from build123d import *

# Parameters (mm, degrees)
SKETCH_1_R               = 11
SKETCH_1_R_2             = 4
EXTRUDE_1_DEPTH          = 7
SKETCH_2_R               = 12
SKETCH_2_R_2             = 10
CUT_EXTRUDE_1_DEPTH      = 0.5
CUT_EXTRUDE_1_DEPTH_BACK = 0.5


with BuildPart() as part:
    # 草图1 → 凸台-拉伸1 (new body)
    with BuildSketch(Plane(origin=(0, 0, 0), x_dir=(1, 0, 0), z_dir=(0, 1, 0))):
        Circle(SKETCH_1_R)
        Circle(SKETCH_1_R_2, mode=Mode.SUBTRACT)
    extrude(amount=EXTRUDE_1_DEPTH)

    # 草图2 → 切除-拉伸1 (cut, two sides)
    with BuildSketch(Plane(origin=(0, 3.5, 0), x_dir=(1, 0, 0), z_dir=(0, 1, 0))) as cut_extrude_1_sk:
        Circle(SKETCH_2_R)
        Circle(SKETCH_2_R_2, mode=Mode.SUBTRACT)
    extrude(amount=CUT_EXTRUDE_1_DEPTH, mode=Mode.SUBTRACT)
    extrude(cut_extrude_1_sk.sketch, amount=-CUT_EXTRUDE_1_DEPTH_BACK, mode=Mode.SUBTRACT)


solid = part.part
Model file for the job. Use its own axes, mm. A direction names the side the tool comes from. Give positions to 0.01 mm unless a question says otherwise; leave off trailing zeros. Write each loop counter-clockwise with the first axis right and the second up, starting at its lowest first coordinate (ties: lowest second). Pieces come first, ordered by that corner, then holes. Notation, with made-up numbers: M -38,-12 L 12,-12 A28 cw 12,25 Z; hole C 32.25,85.5 d10. An arc over 180 degrees is marked long. One line per item, written item: value. Start each with the question number.
Q1. Saw through at A-A, the plane x = 0. Write the cut outline in (y, z), plus the area to 3 significant figures.
Q2. Saw through at B-B, the plane z = 0. Write the cut outline in (x, y).
Q3. Two-plate mould, pull along X, no slides. Class faces 1 (the flat face through (0, 7, 5)), 2 (the cylindrical face through (-2.38, 1.48, 10.74)), 3 (the cylindrical face through (-0.867, 3.451, 3.905)): +X half, -X half, draft (parallel to the pull), parting line (faces both ways), or undercut.
Q4. Saw through at C-C, the plane y = 2. Write the cut outline in (x, z).
Q5. 3-axis set-ups, long thin cutter, end or side, ignore diameter. For faces 4 (the cylindrical face through (-2.38, 5.48, 10.74)), 5 (the flat face through (2, 4, 10)): which of +Z, -Z, +X, -X, +Y, -Y reach the whole face in a straight line?
Q6. Probe probe 1 along X at (y, z) = (2.75, 0); probe 2 along X at (y, z) = (3.5, 0); probe 3 along Y at (x, z) = (2.75, -10). List the from-to ranges inside material, lowest first. Write a range as [from, to].
Q7. Drop flat-ended pins along their axis: pin 1 Ø11 at (x, z) = (0, 0.5) entering from +Y; pin 2 Ø1 at (x, y) = (3.5, 4) entering from -Z; pin 3 Ø1 at (x, y) = (8.5, 0.5) entering from +Z; pin 4 Ø1 at (y, z) = (5.5, 4.5) entering from -X. Give the stop position or say it passes through.
Q8. Saw through at D-D, the plane z = 5.5. Write the cut outline in (x, y).
Output values:
1. outline: M 0,-11 L 3,-11 L 3,-10 L 4,-10 L 4,-11 L 7,-11 L 7,-4 L 0,-4 Z; M 0,4 L 7,4 L 7,11 L 4,11 L 4,10 L 3,10 L 3,11 L 0,11 Z
1. area: 96.0 mm²
2. outline: M -11,0 L -4,0 L -4,7 L -11,7 L -11,4 L -10,4 L -10,3 L -11,3 Z; M 4,0 L 11,0 L 11,3 L 10,3 L 10,4 L 11,4 L 11,7 L 4,7 Z
3. face 1: draft
3. face 2: parting line
3. face 3: undercut
4. outline: C 0,0 d22; hole C 0,0 d8
5. face 4: +Y, -Y
5. face 5: none
6. probe 1: x = [-11, -4], [4, 11]
6. probe 2: x = [-10, -4], [4, 10]
6. probe 3: y = [0, 3], [4, 7]
7. pin 1: stops at y = 7
7. pin 2: stops at z = -10.58
7. pin 3: stops at z = 7.55
7. pin 4: stops at x = -10.25
8. outline: M -9.53,0 L 9.53,0 L 9.53,3 L 8.35,3 L 8.35,4 L 9.53,4 L 9.53,7 L -9.53,7 L -9.53,4 L -8.35,4 L -8.35,3 L -9.53,3 Z
